Verification items for the finished model (mm, model axes). A direction names the side the tool comes from. Coordinates: 2 decimals unless noted, no trailing zeros. Loops run counter-clockwise (first coordinate to the right, second up) from the corner with the lowest first, then second, coordinate; pieces in that order, holes last. Notation, with made-up numbers: (66.5, 0.5) - (96.5, 0.5) arc R13 ccw to (96.5, 8.5) - close; hole circle Ø8 at (85.25, -27.5). An arc over 180 degrees is marked (long way). One line per item, written item: value. Start each with the question number.
(1) Gauge pin test, flat ends, axial feed: P1, Ø1.6, axis at x = 22.5, z = 5.5, coming from the -Y side; P2, Ø3, axis at x = 5.5, z = 3, coming from the -Y side; P3, Ø0.6, axis at x = 22, z = 5, coming from the +Y side. Record the tip position at first contact, or that the pin passes through.
(2) Thickness scan on probe 1 along Y at (x, z) = (11, 0.65); probe 2 along Y at (x, z) = (20, 2.6); probe 3 along Y at (x, z) = (-4, 0.9). Record the ranges inside material, lowest first. Write a range as [from, to].
(3) Section check B-B (x = 9). Record the boundary of the cut face in (y, z), plus the area to 3 significant figures.
(4) Draft check along X on faces 1 (the face through (6.72, -4.31, 2.03)), 2 (the face through (0, -2.5, 0.4)), 3 (the face through (5, 0.5, 3)), 4 (the face through (0, 2.5, 4)). Enter one of: +X half, -X half, draft (parallel to the pull), parting line (faces both ways), or undercut.
(5) Section check C-C (y = 0). Record the boundary of the cut face in (x, z).
(6) Section check A-A (z = 5.3). Record the boundary of the cut face in (x, y).
(7) Set-up check for faces 5 (the face through (0, -1, 0.762)), 6 (the face through (0, -2.5, 4)), 7 (the face through (22, 2, 5)), 8 (the face through (26, 0, 5)): record each of +Z, -Z, +X, -X, +Y, -Y from which the full face is reachable in a straight line by a thin tool's end or side.
(8) Section check D-D (z = 3.6). Record the boundary of the cut face in (x, y), plus the area to 3 significant figures.
```python
from build123d import *
from build123d.topology import SkipClean

# Parameters (mm, degrees)
BOSS_EXTRUDE1_DEPTH = 6
FILLET1_R           = 4
CUT_EXTRUDE1_DEPTH  = 2
SKETCH3_R           = 1.5
SKETCH3_R_2         = 2.5
CUT_EXTRUDE2_DEPTH  = 30.601520231
CUT_EXTRUDE3_DEPTH  = 30.601520231
BOSS_EXTRUDE2_START = -1.27
BOSS_EXTRUDE2_DEPTH = 1.27


with BuildPart() as part:
    # Sketch1 → Boss-Extrude1 (new body)
    with BuildSketch(Plane.XY):
        with BuildLine():
            Line((6.34428877, 4), (24, 4))
            ThreePointArc((24, 4), (28, 0), (24, -4))
            Line((24, -4), (6.34428877, -4))
            ThreePointArc((6.34428877, -4), (-7.5, 0), (6.34428877, 4))
        make_face()
    extrude(amount=BOSS_EXTRUDE1_DEPTH)

    # Fillet1
    fillet1_edges = [part.edges().sort_by_distance(p)[0] for p in [
        (6.34428877, 4, 3),
        (6.34428877, -4, 3),
    ]]
    fillet(fillet1_edges, radius=FILLET1_R)

    # Sketch2 → Cut-Extrude1 (cut)
    with SkipClean():  # the faces are left unmerged after this step: merging them gives an invalid solid
        with BuildSketch(Plane.XY.offset(6)):
            with BuildLine():
                Line((8.261355821, -4), (24, -4))
                ThreePointArc((24, -4), (28, 0), (24, 4))
                Line((24, 4), (8.261355821, 4))
                ThreePointArc((8.261355821, 4), (6.700976826, 4.316901116), (5.387840753, 5.217391304))
                ThreePointArc((5.387840753, 5.217391304), (7.5, 0), (5.387840753, -5.217391304))
                ThreePointArc((5.387840753, -5.217391304), (6.700976826, -4.316901116), (8.261355821, -4))
            make_face()
            with BuildLine():
                Line((20, 2), (24, 2))
                ThreePointArc((24, 2), (26, 0), (24, -2))
                Line((24, -2), (20, -2))
                ThreePointArc((20, -2), (18, 0), (20, 2))
            make_face(mode=Mode.SUBTRACT)
        extrude(amount=-CUT_EXTRUDE1_DEPTH, mode=Mode.SUBTRACT)

    # Sketch3 → Cut-Extrude2 (cut, through all)
    with SkipClean():  # the faces are left unmerged after this step: merging them gives an invalid solid
        with BuildSketch(Plane.XY.offset(6)):
            with Locations((20, 0)):
                Circle(SKETCH3_R)
            with Locations((24, 0)):
                Circle(SKETCH3_R)
            Circle(SKETCH3_R_2)
        extrude(amount=-CUT_EXTRUDE2_DEPTH, mode=Mode.SUBTRACT)

    # Sketch4 → Cut-Extrude3 (cut, through all)
    with SkipClean():  # the faces are left unmerged after this step: merging them gives an invalid solid
        with BuildSketch(Plane.XY.offset(6)):
            with BuildLine():
                Line((-8.079422864, 0.5), (8.133974596, 0.5))
                ThreePointArc((8.133974596, 0.5), (10, 0), (8.133974596, -0.5))
                Line((8.133974596, -0.5), (-8.079422864, -0.5))
                Line((-8.079422864, -0.5), (-8.079422864, 0.5))
            make_face()
        extrude(amount=-CUT_EXTRUDE3_DEPTH, mode=Mode.SUBTRACT)

    # Sketch5 → Boss-Extrude2 (add)
    with SkipClean():  # the faces are left unmerged after this step: merging them gives an invalid solid
        with BuildSketch(Plane(origin=(0, 0, 0.762), x_dir=(-1, 0, 0), z_dir=(0, 0, -1)).offset(BOSS_EXTRUDE2_START)):
            with BuildLine():
                Line((-2.449489743, 0.5), (-0.656848727, 0.5))
                ThreePointArc((-0.656848727, 0.5), (0, 0.8255), (0.656848727, 0.5))
                Line((0.656848727, 0.5), (2.449489743, 0.5))
                ThreePointArc((2.449489743, 0.5), (0, 2.5), (-2.449489743, 0.5))
            make_face()
            with BuildLine():
                Line((-2.449489743, -0.5), (-0.656848727, -0.5))
                ThreePointArc((-0.656848727, -0.5), (0, -0.8255), (0.656848727, -0.5))
                Line((0.656848727, -0.5), (2.449489743, -0.5))
                ThreePointArc((2.449489743, -0.5), (0, -2.5), (-2.449489743, -0.5))
            make_face()
        extrude(amount=BOSS_EXTRUDE2_DEPTH)


solid = part.part
```
Responses:
1. P1: stops at y = -2
1. P2: stops at y = -6.34
1. P3: stops at y = 2
2. probe 1: y = [-4, 4]
2. probe 2: y = [-4, -1.5], [1.5, 4]
2. probe 3: y = [-6.34, -0.5], [0.5, 6.34]
3. outline: (-4, 0) - (-1, 0) - (-1, 4) - (-4, 4) - close; (1, 0) - (4, 0) - (4, 4) - (1, 4) - close
3. area: 24.0 mm²
4. face 1: +X half
4. face 2: undercut
4. face 3: draft
4. face 4: undercut
5. outline: (10, 0) - (18.5, 0) - (18.5, 6) - (18, 6) - (18, 4) - (10, 4) - close; (21.5, 0) - (22.5, 0) - (22.5, 6) - (21.5, 6) - close; (25.5, 0) - (28, 0) - (28, 4) - (26, 4) - (26, 6) - (25.5, 6) - close
6. outline: (-7.48, -0.5) arc R7.5 ccw to (7.48, -0.5) - (2.45, -0.5) arc R2.5 cw to (-2.45, -0.5) - close; (-7.48, 0.5) - (-2.45, 0.5) arc R2.5 cw to (2.45, 0.5) - (7.48, 0.5) arc R7.5 ccw to start; (20, -2) - (24, -2) arc R2 ccw to (24, 2) - (20, 2) arc R2 ccw to start; hole circle Ø3 at (20, 0); hole circle Ø3 at (24, 0)
7. face 5: -Z
7. face 6: +Z
7. face 7: +Z, +X, +Y
7. face 8: +Z, +X
8. outline: (-7.48, -0.5) arc R7.5 ccw to (5.39, -5.22) arc R4 cw to (8.26, -4) - (24, -4) arc R4 ccw to (24, 4) - (8.26, 4) arc R4 cw to (5.39, 5.22) arc R7.5 ccw to (-7.48, 0.5) - (-2.45, 0.5) arc R2.5 cw to (2.45, 0.5) - (8.13, 0.5) arc R1 cw (long way) to (8.13, -0.5) - (2.45, -0.5) arc R2.5 cw to (-2.45, -0.5) - close; hole circle Ø3 at (20, 0); hole circle Ø3 at (24, 0)
8. area: 290 mm²
